Input: part model. Units: mm. Frame: model coordinates. A direction names the side the tool comes from. Round coordinates to 2 decimals unless told otherwise and drop trailing zeros. Loops run counter-clockwise (first coordinate to the right, second up) from the corner with the lowest first, then second, coordinate; pieces in that order, holes last. Notation, with made-up numbers: (84, 74) - (93, 74) arc R10 ccw to (93, 88) - close; hole circle Ø11 at (-20.75, 57.25). An arc over 180 degrees is marked (long way). One line per question, with ' | ' between items. Start each with the question number.
Item 1: Section B-B, the plane z = -15. Return loops of the section in (x, y).
Item 2: Draft query along Z for faces 1 (the face through (24, 14, -23)), 2 (the face through (8, 2, -39)), 3 (the face through (0.6, 0.57, -29.41)), 4 (the face through (26.699, 7.605, -0.285)). Return one class per face: pulls with the +Z half, pulls with the -Z half, needs draft (parallel to the pull), parting line crosses it, or undercut.
Item 3: Section C-C, the plane x = 24.5. Return loops of the section in (y, z).
Item 4: Material intervals for line 1 along Y through (x, z) = (2.5, -46.5); line 2 along Y through (x, z) = (24.5, -12.25); line 3 along X through (y, z) = (2.25, -41.5), sorted ascending.
Item 5: Set-up query: faces 5 (the face through (22.2, 15, -11.7)), 6 (the face through (1, 15, -15)), 7 (the face through (1.5, 13.6, -55)), 8 (the face through (23, 7, -8)). Return all of +Z, -Z, +X, -X, +Y, -Y with unobstructed straight access to the full face (end or side cutting, diameter ignored); none if empty.
Item 6: Section A-A, the plane y = 7.35. Return loops of the section in (x, z), plus the area to 3 significant figures.
Item 7: First-contact query: pin 1 (0.9 mm diameter, centred on y = 1, z = -41.5, fed in from -X); pin 2 (1.5 mm diameter, centred on x = 25, y = 13.5, fed in from -Z); pin 3 (0.9 mm diameter, centred on x = 1, z = -38.5, fed in from -Y). Flat tips, straight axial feed; report the tip coordinate or a pass-through.
Item 8: Section D-D, the plane z = -5.5. Return loops of the section in (x, y), plus the area to 3 significant figures.
```python
from build123d import *

# Parameters (mm, degrees)
BOSS_EXTRUDE1_DEPTH = 3
SKETCH2_R           = 1.25
SKETCH2_W           = 12.45
SKETCH2_H           = 22.7
CUT_EXTRUDE1_DEPTH  = 3
SKETCH3_W           = 3
SKETCH3_H           = 58
BOSS_EXTRUDE2_DEPTH = 15
BOSS_EXTRUDE3_DEPTH = 12
FILLET1_R           = 2
FILLET2_R           = 2
FILLET3_R           = 1
CUT_EXTRUDE2_DEPTH  = 3
SKETCH7_R           = 1.55
CUT_EXTRUDE3_DEPTH  = 48.728398255


with BuildPart() as part:
    # Sketch1 → Boss-Extrude1 (new body)
    with BuildSketch(Plane(origin=(0, 0, 0), x_dir=(1, 0, 0), z_dir=(0, 1, 0))):
        with BuildLine():
            Line((27, 8), (20, 8))
            ThreePointArc((20, 8), (17.5, 5.5), (20, 3))
            Line((20, 3), (27, 3))
            Line((27, 3), (27, 0))
            Line((27, 0), (0, 0))
            Line((0, 0), (0, 58))
            Line((0, 58), (27, 58))
            Line((27, 58), (27, 8))
        make_face()
    extrude(amount=BOSS_EXTRUDE1_DEPTH)

    # Sketch2 → Cut-Extrude1 (cut)
    with BuildSketch(Plane(origin=(0, 3, 0), x_dir=(1, 0, 0), z_dir=(0, 1, 0))):
        with Locations(Location((14.225, 53.1, 0), (0, 0, 270))):
            Circle(SKETCH2_R)
        with Locations(Location((14.225, 25.6, 0), (0, 0, 270))):
            Circle(SKETCH2_R)
        with Locations((14.225, 39.35)):
            Rectangle(SKETCH2_W, SKETCH2_H)
    extrude(amount=-CUT_EXTRUDE1_DEPTH, mode=Mode.SUBTRACT)

    # Sketch3 → Boss-Extrude2 (add)
    with BuildSketch(Plane(origin=(0, 3, 0), x_dir=(1, 0, 0), z_dir=(0, 1, 0))):
        with Locations((1.5, 29)):
            Rectangle(SKETCH3_W, SKETCH3_H)
    extrude(amount=BOSS_EXTRUDE2_DEPTH)

    # Sketch4 → Boss-Extrude3 (add)
    with BuildSketch(Plane(origin=(0, 3, 0), x_dir=(1, 0, 0), z_dir=(0, 1, 0))):
        with BuildLine():
            Line((20, 11), (22, 11))
            Line((22, 11), (22, 23))
            Line((22, 23), (27, 23))
            Line((27, 23), (27, 11))
            Line((27, 11), (27, 8))
            Line((27, 8), (20, 8))
            ThreePointArc((20, 8), (17.5, 5.5), (20, 3))
            Line((20, 3), (27, 3))
            Line((27, 3), (27, 0))
            Line((27, 0), (20, 0))
            ThreePointArc((20, 0), (14.5, 5.5), (20, 11))
        make_face()
    extrude(amount=BOSS_EXTRUDE3_DEPTH)

    # Fillet1
    fillet1_edges = [part.edges().sort_by_distance(p)[0] for p in [
        (0, 0, -29),
        (3, 3, -29),
    ]]
    fillet(fillet1_edges, radius=FILLET1_R)

    # Fillet2
    fillet2_edges = [part.edges().sort_by_distance(p)[0] for p in [
        (1.5, 18, 0),
        (1.5, 18, -58),
    ]]
    fillet(fillet2_edges, radius=FILLET2_R)

    # Fillet3
    fillet3_edges = [part.edges().sort_by_distance(p)[0] for p in [
        (27, 1.5, -58),
        (27, 7.5, -8),
        (27, 7.5, -3),
        (27, 7.5, 0),
        (27, 9, -23),
        (22, 9, -23),
    ]]
    fillet(fillet3_edges, radius=FILLET3_R)

    # Sketch5 → Cut-Extrude2 (cut)
    with BuildSketch(Plane.ZY):
        with BuildLine():
            Line((-53.65, 15), (-31.85, 15))
            ThreePointArc((-31.85, 15), (-30.5, 13.65), (-31.85, 12.3))
            Line((-31.85, 12.3), (-53.65, 12.3))
            ThreePointArc((-53.65, 12.3), (-55, 13.65), (-53.65, 15))
        make_face()
        with BuildLine():
            Line((-53.65, 8.7), (-31.85, 8.7))
            ThreePointArc((-31.85, 8.7), (-30.5, 7.35), (-31.85, 6))
            Line((-31.85, 6), (-53.65, 6))
            ThreePointArc((-53.65, 6), (-55, 7.35), (-53.65, 8.7))
        make_face()
        with BuildLine():
            Line((-26.15, 15), (-4.35, 15))
            ThreePointArc((-4.35, 15), (-3, 13.65), (-4.35, 12.3))
            Line((-4.35, 12.3), (-26.15, 12.3))
            ThreePointArc((-26.15, 12.3), (-27.5, 13.65), (-26.15, 15))
        make_face()
        with BuildLine():
            Line((-26.15, 8.7), (-4.35, 8.7))
            ThreePointArc((-4.35, 8.7), (-3, 7.35), (-4.35, 6))
            Line((-4.35, 6), (-26.15, 6))
            ThreePointArc((-26.15, 6), (-27.5, 7.35), (-26.15, 8.7))
        make_face()
    extrude(amount=-CUT_EXTRUDE2_DEPTH, mode=Mode.SUBTRACT)

    # Sketch7 → Cut-Extrude3 (cut, through all)
    with BuildSketch(Plane(origin=(0, 0, -23), x_dir=(-1, 0, 0), z_dir=(0, 0, -1))):
        with Locations(Location((-24.5, 11, 0), (0, 0, 165.407449398))):
            Circle(SKETCH7_R)
    extrude(amount=-CUT_EXTRUDE3_DEPTH, mode=Mode.SUBTRACT)


solid = part.part
```
Return value:
1) outline: (0, 2) arc R2 ccw to (2, 0) - (27, 0) - (27, 15) - (22, 15) - (22, 3) - (5, 3) arc R2 cw to (3, 5) - (3, 6) - (0, 6) - close; (0, 8.7) - (3, 8.7) - (3, 12.3) - (0, 12.3) - close; (0, 15) - (3, 15) - (3, 18) - (0, 18) - close; hole circle Ø3.1 at (24.5, 11)
2) face 1: pulls with the -Z half | face 2: undercut | face 3: needs draft | face 4: pulls with the +Z half
3) outline: (0, -58) - (3, -58) - (3, -23) - (9.45, -23) - (9.45, -8) - (0, -8) - close; (0, -3) - (9.45, -3) - (9.45, 0) - (0, 0) - close; (12.55, -23) - (15, -23) - (15, -8) - (12.55, -8) - close; (12.55, -3) - (15, -3) - (15, 0) - (12.55, 0) - close
4) line 1: 0 to 6, 8.7 to 12.3, 15 to 18 | line 2: 0 to 9.45, 12.55 to 15 | line 3: 0 to 8, 20.45 to 27
5) face 5: +Z, -Z, +X, +Y | face 6: -X | face 7: +X, -X | face 8: +X, +Y, -Y
6) outline: (0, -58) - (3, -58) - (3, -55) - (0, -55) - close; (0, -30.5) - (3, -30.5) - (3, -27.5) - (0, -27.5) - close; (0, -3) - (3, -3) - (3, 0) - (0, 0) - close; (20, -11) - (22, -11) - (22, -22) arc R1 ccw to (23, -23) - (26, -23) arc R1 ccw to (27, -22) - (27, -9) arc R1 ccw to (26, -8) - (20, -8) arc R2.5 cw to (20, -3) - (26, -3) arc R1 ccw to (27, -2) - (27, -1) arc R1 ccw to (26, 0) - (20, 0) arc R5.5 ccw to start | area: 166 mm2
7) pin 1: x = 0.08 | pin 2: z = -23 | pin 3: y = 0.08
8) outline: (0, 2) arc R2 ccw to (2, 0) - (17.5, 0) - (17.5, 15) - (14.5, 15) - (14.5, 3) - (5, 3) arc R2 cw to (3, 5) - (3, 6) - (0, 6) - close; (0, 8.7) - (3, 8.7) - (3, 12.3) - (0, 12.3) - close; (0, 15) - (3, 15) - (3, 18) - (0, 18) - close | area: 117 mm2
